from build123d import *

# Parameters (mm, degrees)
SKETCH1_W           = 25
SKETCH1_H           = 50
SKETCH1_R           = 3.4
BOSS_EXTRUDE1_DEPTH = 3
SKETCH2_W           = 50
SKETCH2_H           = 3
BOSS_EXTRUDE2_DEPTH = 8
SKETCH3_W           = 8
SKETCH3_H           = 50
BOSS_EXTRUDE3_DEPTH = 42
SKETCH4_R           = 2.65
CUT_EXTRUDE1_DEPTH  = 0.5
SKETCH5_R           = 5.888972746
CUT_EXTRUDE2_DEPTH  = 9
FILLET2_R           = 1
SKETCH6_R           = 12.6
BOSS_EXTRUDE4_DEPTH = 2
FILLET4_R           = 1
SKETCH8_R           = 1.589780168
SKETCH8_R_2         = 1.777428262
CUT_EXTRUDE3_DEPTH  = 10
SKETCH9_W           = 49.021678163
SKETCH9_H           = 20.976854622
CUT_EXTRUDE4_DEPTH  = 68.79439129
SKETCH11_R          = 2.1
CUT_EXTRUDE5_DEPTH  = 59.480168703
SKETCH14_R          = 2.6
CUT_EXTRUDE6_DEPTH  = 0.5


with BuildPart() as part:
    # Sketch1 → Boss-Extrude1 (new body)
    with BuildSketch(Plane(origin=(0, 0, 0), x_dir=(1, 0, 0), z_dir=(0, 1, 0))):
        with Locations((2.276951673, 11.384758364)):
            Rectangle(SKETCH1_W, SKETCH1_H)
        with Locations(Location((1.276951673, 11.384758364, 0), (0, 0, 270))):
            Circle(SKETCH1_R, mode=Mode.SUBTRACT)
    extrude(amount=BOSS_EXTRUDE1_DEPTH)

    # Sketch2 → Boss-Extrude2 (add)
    with BuildSketch(Plane.ZY.offset(10.223048327)):
        with Locations((-11.384758364, 1.5)):
            Rectangle(SKETCH2_W, SKETCH2_H)
    extrude(amount=BOSS_EXTRUDE2_DEPTH)

    # Sketch3 → Boss-Extrude3 (add)
    with BuildSketch(Plane.XZ):
        with Locations((-14.223048327, -11.384758364)):
            Rectangle(SKETCH3_W, SKETCH3_H)
    extrude(amount=BOSS_EXTRUDE3_DEPTH)

    # Sketch4 → Cut-Extrude1 (cut)
    with BuildSketch(Plane(origin=(0, 3, 0), x_dir=(1, 0, 0), z_dir=(0, 1, 0))):
        with Locations(Location((-14.223048327, 32.384758364, 0), (0, 0, 270))):
            Circle(SKETCH4_R)
        with Locations(Location((-14.223048327, -9.615241636, 0), (0, 0, 270))):
            Circle(SKETCH4_R)
    cut_extrude1 = extrude(amount=-CUT_EXTRUDE1_DEPTH, mode=Mode.SUBTRACT)

    # Mirror1: Cut-Extrude1 across plane
    add(cut_extrude1.mirror(Plane.ZX.offset(-19.5)), mode=Mode.SUBTRACT)

    # Sketch5 → Cut-Extrude2 (cut)
    with BuildSketch(Plane.ZY.offset(18.223048327)):
        with Locations((-11.836279124, -21)):
            Circle(SKETCH5_R)
    extrude(amount=-CUT_EXTRUDE2_DEPTH, mode=Mode.SUBTRACT)

    # Fillet2
    fillet2_edges = [part.edges().sort_by_distance(p)[0] for p in [
        (-10.223048327, -21, -17.72525187),
    ]]
    fillet(fillet2_edges, radius=FILLET2_R)

    # Mirror2: Cut-Extrude1 across plane
    add(cut_extrude1.mirror(Plane.ZY.offset(1.723048327)), mode=Mode.SUBTRACT)

    # Sketch6 → Boss-Extrude4 (add)
    with BuildSketch(Plane(origin=(0, 3, 0), x_dir=(1, 0, 0), z_dir=(0, 1, 0))):
        with BuildLine():
            Line((14.776951673, 5.825082115), (14.776951673, 16.944434614))
            ThreePointArc((14.776951673, 16.944434614), (-13.323048327, 11.384758364), (14.776951673, 5.825082115))
        make_face()
        with Locations(Location((1.276951673, 11.384758364, 0), (0, 0, 270))):
            Circle(SKETCH6_R, mode=Mode.SUBTRACT)
    extrude(amount=BOSS_EXTRUDE4_DEPTH)

    # Fillet4
    # the kernel refuses this fillet: 1 mm, written as the material it takes off along each edge
    with BuildSketch(Plane(origin=(14.776951673, 5, -3.325082115), x_dir=(0, -1, 0), z_dir=(0, 0, -1))) as fillet4_piece_1:
        with BuildLine():
            CenterArc((FILLET4_R, FILLET4_R), FILLET4_R, 180, 90)
            Line((0, FILLET4_R), (0, 0))
            Line((0, 0), (FILLET4_R, 0))
        make_face()
    extrude(amount=16.119352499, mode=Mode.SUBTRACT)

    # Sketch8 → Cut-Extrude3 (cut)
    with BuildSketch(Plane(origin=(0, 3, 0), x_dir=(1, 0, 0), z_dir=(0, 1, 0))):
        with Locations(Location((1.276951673, 19.884758364, 0), (0, 0, 270))):
            Circle(SKETCH8_R)
        with Locations(Location((1.276951673, 2.884758364, 0), (0, 0, 270))):
            Circle(SKETCH8_R_2)
    extrude(amount=-CUT_EXTRUDE3_DEPTH, mode=Mode.SUBTRACT)

    # Sketch9 → Cut-Extrude4 (cut, through all)
    with BuildSketch(Plane.XY.offset(13.615241636)):
        with Locations((-9.733887409, 10.488427311)):
            Rectangle(SKETCH9_W, SKETCH9_H)
    extrude(amount=-CUT_EXTRUDE4_DEPTH, mode=Mode.SUBTRACT)

    # Sketch11 → Cut-Extrude5 (cut, through all)
    with BuildSketch(Plane(origin=(0, 0, 0), x_dir=(1, 0, 0), z_dir=(0, 1, 0))):
        with Locations(Location((-14.223048327, 32.384758364, 0), (0, 0, 270))):
            Circle(SKETCH11_R)
    cut_extrude5 = extrude(amount=-CUT_EXTRUDE5_DEPTH, mode=Mode.SUBTRACT)

    # Mirror3: Cut-Extrude5 across plane
    add(cut_extrude5.mirror(Plane.XY.offset(-11.384758364)), mode=Mode.SUBTRACT)

    # Sketch14 → Cut-Extrude6 (cut)
    with BuildSketch(Plane(origin=(0, 0, 0), x_dir=(1, 0, 0), z_dir=(0, 1, 0))):
        with Locations(Location((-14.223048327, -9.615241636, 0), (0, 0, 270))):
            Circle(SKETCH14_R)
    cut_extrude6 = extrude(amount=-CUT_EXTRUDE6_DEPTH, mode=Mode.SUBTRACT)

    # Mirror4: Cut-Extrude6 across plane
    add(cut_extrude6.mirror(Plane.XY.offset(-11.384758364)), mode=Mode.SUBTRACT)


solid = part.part
Input: part model. Units: mm. Frame: model coordinates. A direction names the side the tool comes from. Give positions to 0.01 mm unless a question says otherwise; leave off trailing zeros. Order: outer loops, then holes, each group sorted by start corner. A loop starts at its lowest first (then second) coordinate and runs counter-clockwise, first axis right, second up. Notation, with made-up numbers: (84.25, -5.5) - (121.25, -5.5) arc R28 cw to (121.25, 21.5) - close; hole circle Ø6 at (-26.75, 18.25). An arc over 180 degrees is marked (long way). Answer as a JSON object with one key per item and string values. Group by question number.
Q1. Cut plane A-A, the plane y = -21. Output: boundary loops of the cut face in (x, z).
Q2. Mould query, pull axis X, two halves, no side actions, for faces 4 (the face through (-10.223, -16, -17)), 5 (the face through (-14, -21, 13.615)), 6 (the face through (-11.596, -41.754, 9.27)). Classes: pulls with the +X half, pulls with the -X half, needs draft (parallel to the pull), parting line crosses it, or undercut.
Q3. Set-up query: faces 1 (the face through (-12, -0.5, -33)), 2 (the face through (-18.223, -16, -17)), 3 (the face through (-12, -41.5, 9)). Return all of +Z, -Z, +X, -X, +Y, -Y with unobstructed straight access to the full face (end or side cutting, diameter ignored); none if empty.
Q4. Cut plane C-C, the plane x = -17.5. Output: boundary loops of the cut face in (y, z), then the cut area to 3 significant figures.
Q5. Line query: probe 1 along Z at (x, y) = (-14, -9.5); probe 2 along Z at (x, y) = (-13.25, -14); probe 3 along Z at (x, y) = (-16.75, -19.5). Output: solid intervals per line, ascending.
Q6. Cut plane B-B, the plane x = -15. Count the separate pieces of the cut face and the enclosed holes in it, then the cut area to 3 significant figures.
Q7. First-contact query: pin 1 Ø4 at (x, z) = (-14.5, -32) entering from +Y; pin 2 Ø1.6 at (x, z) = (-13, 8.5) entering from -Y. Flat tips, straight axial feed; report the tip coordinate or a pass-through.
Q8. Cut plane D-D, the plane y = -29. Output: boundary loops of the cut face in (x, z).
Results:
{
 "1": {"outline": "(-18.22, -36.38) - (-10.22, -36.38) - (-10.22, -18.73) arc R1 ccw to (-11.22, -17.73) - (-18.22, -17.73) - close; (-18.22, -5.95) - (-11.22, -5.95) arc R1 ccw to (-10.22, -4.95) - (-10.22, 13.62) - (-18.22, 13.62) - close; hole circle Ø4.2 at (-14.22, -32.38); hole circle Ø4.2 at (-14.22, 9.62)"},
 "2": {"face 4": "pulls with the +X half", "face 5": "needs draft", "face 6": "undercut"},
 "3": {"face 1": "+Y", "face 2": "+Z, -Z, -X, +Y, -Y", "face 3": "-Y"},
 "4": {"outline": "(-42, -36.38) - (0, -36.38) - (0, 13.62) - (-42, 13.62) - close; hole circle Ø11.78 at (-21, -11.84)", "area": "1,990 mm^2"},
 "5": {"probe 1": "-36.38 to -34.47, -30.3 to 7.53, 11.7 to 13.62", "probe 2": "-36.38 to -34.25, -30.52 to 7.75, 11.48 to 13.62", "probe 3": "-36.38 to -17.53, -6.14 to 13.62"},
 "6": {"separate pieces": "3", "enclosed holes": "1", "area": "1,660 mm^2"},
 "7": {"pin 1": "y = -0.5", "pin 2": "y = -41.5"},
 "8": {"outline": "(-18.22, -36.38) - (-10.22, -36.38) - (-10.22, 13.62) - (-18.22, 13.62) - close; hole circle Ø4.2 at (-14.22, -32.38); hole circle Ø4.2 at (-14.22, 9.62)"}
}
